Source: CAD feature listing. Evaluate the final solid. Frame: model axes, mm. Give positions to 0.01 mm unless a question says otherwise; leave off trailing zeros. Loops run counter-clockwise (first coordinate to the right, second up) from the corner with the lowest first, then second, coordinate; pieces in that order, holes last. Notation, with made-up numbers: M 69,49.5 L 114,49.5 A9 ccw 114,54.5 Z; hole C -8,-33 d10. An arc over 180 degrees is marked long. Answer in a Markdown table with one row per item.
```python
from build123d import *

# Parameters (mm, degrees)
ENL_V_MAT_EXTRU_1_DEPTH = 1


with BuildPart() as part:
    # Esquisse2 → Révolution2 (revolve)
    with BuildSketch(Plane.XY):
        with BuildLine():
            Line((-1.5, -3), (-1.5, -6))
            Line((-1.5, -6), (-4, -6))
            Line((-4, -6), (-4, 0))
            ThreePointArc((-4, 0), (-2.828427125, 2.828427125), (0, 4))
            Line((0, 4), (0, -3))
            Line((0, -3), (-1.5, -3))
        make_face()
    revolve(axis=Axis((0, 4, 0), (0, -1, 0)))

    # Esquisse3 → Enlèv. mat.-Extru.1 (cut)
    with BuildSketch(Plane.XZ.offset(6)):
        with BuildLine():
            add(Edge.make_bspline(
                [(-1.80863124, 2.541345123), (-1.808479721, 2.566576945), (-1.808185465, 2.615578129), (-1.805014729, 2.686862301), (-1.799544973, 2.753773198), (-1.792519265, 2.816312807), (-1.782799384, 2.874524095), (-1.771677826, 2.928435828), (-1.75798753, 2.978054639), (-1.741996794, 3.023469068), (-1.724042414, 3.06548569), (-1.704301487, 3.104630802), (-1.682899044, 3.141401404), (-1.659979633, 3.175784688), (-1.634459695, 3.207014642), (-1.607837422, 3.236160804), (-1.579113212, 3.262654216), (-1.548550296, 3.286362241), (-1.516934602, 3.307796564), (-1.483892299, 3.325862839), (-1.450188991, 3.341600286), (-1.415394884, 3.354330516), (-1.379762252, 3.364219477), (-1.343163483, 3.371125489), (-1.305772607, 3.375881264), (-1.280433508, 3.376250629), (-1.267698248, 3.376436269)],
                knots=[0, 0, 0, 0, 1.622528522, 3.151013738, 4.587225782, 5.939257941, 7.196658267, 8.381214254, 9.47772444, 10.503964975, 11.475138444, 12.414102326, 13.321377868, 14.209997518, 15.068075989, 15.912287155, 16.746865696, 17.577313739, 18.397854368, 19.200328723, 19.996378645, 20.787862277, 21.580050128, 22.371504404, 23.181529048, 24, 24, 24, 24], degree=3))
            add(Edge.make_bspline(
                [(-1.267698248, 3.376436269), (-1.253805469, 3.376070417), (-1.226383591, 3.37534829), (-1.185688202, 3.371418433), (-1.146357234, 3.363478815), (-1.107851049, 3.353522224), (-1.070793349, 3.339911348), (-1.034450069, 3.324259466), (-0.999939833, 3.304434891), (-0.966085568, 3.282749499), (-0.934048036, 3.25774196), (-0.903405408, 3.230569518), (-0.875113051, 3.200304639), (-0.848139657, 3.16798873), (-0.823868807, 3.132356169), (-0.800763662, 3.094654654), (-0.780305532, 3.05394524), (-0.760895229, 3.010948076), (-0.74421092, 2.964519866), (-0.729110025, 2.91492575), (-0.716872402, 2.861547844), (-0.706720882, 2.804552033), (-0.698897695, 2.743842361), (-0.693120072, 2.679563038), (-0.690103596, 2.611653966), (-0.689533129, 2.565198361), (-0.689240215, 2.541345123)],
                knots=[0, 0, 0, 0, 0.875057392, 1.727207867, 2.570264412, 3.399251263, 4.229017074, 5.053828049, 5.887584622, 6.731829445, 7.583639997, 8.443960147, 9.308026848, 10.190032267, 11.091770676, 12.020167189, 12.972467704, 13.958579741, 14.989078804, 16.076606933, 17.221320015, 18.435081626, 19.720875061, 21.074561036, 22.497895074, 24, 24, 24, 24], degree=3))
            add(Edge.make_bspline(
                [(-0.689240215, 2.541345123), (-0.689536199, 2.517598254), (-0.690112578, 2.471355268), (-0.693085762, 2.403758625), (-0.699013134, 2.339828893), (-0.706311275, 2.279386639), (-0.716548088, 2.222615428), (-0.729012582, 2.169485269), (-0.742990504, 2.11971682), (-0.760077838, 2.073746258), (-0.778998468, 2.030799872), (-0.799526075, 1.99045447), (-0.822133943, 1.952630546), (-0.847166636, 1.917738486), (-0.873431331, 1.884680376), (-0.902069059, 1.854605169), (-0.93255791, 1.826939612), (-0.96482414, 1.802036036), (-0.998498431, 1.779578013), (-1.033792029, 1.760620727), (-1.069815262, 1.743794249), (-1.107372434, 1.731042265), (-1.145702223, 1.720159494), (-1.185450047, 1.713129804), (-1.226246928, 1.70847555), (-1.253798722, 1.707844413), (-1.267698248, 1.707526012)],
                knots=[0, 0, 0, 0, 1.496607488, 2.914388442, 4.262485651, 5.541812885, 6.749953981, 7.895567619, 8.980172623, 10.005210728, 10.983286874, 11.936336572, 12.856292636, 13.757107149, 14.640766483, 15.514956722, 16.370989637, 17.232841377, 18.081413197, 18.918442167, 19.755471137, 20.583656588, 21.41504191, 22.264086897, 23.124254193, 24, 24, 24, 24], degree=3))
            add(Edge.make_bspline(
                [(-1.267698248, 1.707526012), (-1.28053559, 1.707744144), (-1.305960862, 1.708176169), (-1.343505356, 1.712413318), (-1.38007908, 1.719445505), (-1.415574616, 1.729301415), (-1.450241362, 1.741814634), (-1.483928981, 1.756972649), (-1.516416052, 1.775327151), (-1.54801261, 1.795949979), (-1.578259763, 1.819406928), (-1.6064329, 1.845919153), (-1.633209394, 1.874853048), (-1.658058785, 1.906520629), (-1.68153021, 1.940717467), (-1.70268935, 1.977765743), (-1.722416535, 2.017269766), (-1.740706112, 2.059533815), (-1.757219877, 2.105292204), (-1.770391091, 2.155440158), (-1.782811418, 2.209430466), (-1.79192615, 2.267809314), (-1.799834358, 2.33013628), (-1.804422361, 2.396815965), (-1.808343164, 2.467627223), (-1.808533454, 2.51632197), (-1.80863124, 2.541345123)],
                knots=[0, 0, 0, 0, 0.82614074, 1.636230647, 2.42850654, 3.22151677, 4.005075515, 4.799112676, 5.596456327, 6.404618302, 7.226350817, 8.05679228, 8.892237205, 9.761873943, 10.645770802, 11.559890835, 12.505927976, 13.487073095, 14.523090282, 15.633895838, 16.822583925, 18.088023083, 19.435493537, 20.865857947, 22.389433785, 24, 24, 24, 24], degree=3))
        make_face()
        with BuildLine():
            add(Edge.make_bspline(
                [(-1.605105599, 2.541981141), (-1.605023852, 2.520672046), (-1.604865594, 2.479419233), (-1.602515721, 2.419724601), (-1.599170136, 2.364139577), (-1.59416568, 2.312679231), (-1.587492401, 2.265267043), (-1.579593913, 2.22196849), (-1.570588452, 2.182700619), (-1.559609283, 2.147398904), (-1.547452492, 2.115233539), (-1.533935704, 2.085621273), (-1.519900759, 2.057891237), (-1.504090822, 2.032593058), (-1.487347707, 2.00938102), (-1.469369083, 1.988343478), (-1.450796759, 1.969019299), (-1.424302992, 1.947561621), (-1.390356536, 1.925127641), (-1.348216049, 1.905674198), (-1.305758021, 1.892833006), (-1.277113233, 1.891405835), (-1.262928115, 1.890699089)],
                knots=[0, 0, 0, 0, 1.564601651, 3.028951736, 4.386019676, 5.653114642, 6.824348509, 7.900668805, 8.88431448, 9.780488761, 10.613163047, 11.407444027, 12.169849642, 12.89344098, 13.595615509, 14.26934431, 14.924332585, 15.560171042, 16.769153194, 17.901006317, 18.960562374, 20, 20, 20, 20], degree=3))
            add(Edge.make_bspline(
                [(-1.262928115, 1.890699089), (-1.246853522, 1.891540168), (-1.214804369, 1.893217091), (-1.167603677, 1.905427209), (-1.122345984, 1.925920174), (-1.086485855, 1.949072591), (-1.05939208, 1.971591143), (-1.039825463, 1.990761174), (-1.02179068, 2.012163191), (-1.004765256, 2.035471294), (-0.989370848, 2.06106677), (-0.974527097, 2.088368697), (-0.961602786, 2.118032092), (-0.95413322, 2.138702882), (-0.950325451, 2.149240255)],
                knots=[0, 0, 0, 0, 1.331887272, 2.655486065, 4.012646414, 5.436183829, 6.178803566, 6.930724497, 7.703763371, 8.496530827, 9.320959298, 10.178042319, 11.071218497, 12, 12, 12, 12], degree=3))
            add(Edge.make_bspline(
                [(-0.950325451, 2.149240255), (-0.945737968, 2.163084868), (-0.936386065, 2.191308069), (-0.924669416, 2.235249723), (-0.914969473, 2.281357725), (-0.906617281, 2.329386525), (-0.90027545, 2.37957809), (-0.895891912, 2.431884075), (-0.893377451, 2.486304801), (-0.892971987, 2.523216067), (-0.892765856, 2.541981141)],
                knots=[0, 0, 0, 0, 0.877617242, 1.789083553, 2.735016418, 3.71249782, 4.722174671, 5.778575778, 6.870664861, 8, 8, 8, 8], degree=3))
            add(Edge.make_bspline(
                [(-0.892765856, 2.541981141), (-0.892815192, 2.560748136), (-0.892911405, 2.597346919), (-0.895770969, 2.650881984), (-0.899229308, 2.701840221), (-0.905195582, 2.750054281), (-0.911872778, 2.795764776), (-0.921031545, 2.838648534), (-0.930854849, 2.879133664), (-0.943127016, 2.916720139), (-0.956544156, 2.951787091), (-0.970695385, 2.984451245), (-0.985996373, 3.014738738), (-1.002854445, 3.04226954), (-1.020647463, 3.06749779), (-1.039441811, 3.090271765), (-1.05951754, 3.110463274), (-1.087584092, 3.133229632), (-1.123765401, 3.156924472), (-1.169007106, 3.178189343), (-1.215723695, 3.190725625), (-1.247275437, 3.192421751), (-1.262928115, 3.193263192)],
                knots=[0, 0, 0, 0, 1.353201578, 2.638969622, 3.865559904, 5.035676431, 6.141732754, 7.195734042, 8.19695873, 9.144657206, 10.044788335, 10.904062871, 11.710933862, 12.489720227, 13.229995877, 13.935715626, 14.616825307, 15.279494989, 16.538995736, 17.725922936, 18.871840505, 20, 20, 20, 20], degree=3))
            add(Edge.make_bspline(
                [(-1.262928115, 3.193263192), (-1.277109142, 3.192542637), (-1.305847895, 3.191082387), (-1.348370358, 3.178419537), (-1.390359144, 3.158811848), (-1.424078124, 3.13636234), (-1.450352786, 3.114927418), (-1.469178663, 3.096042766), (-1.486571406, 3.074886349), (-1.503356006, 3.051861153), (-1.518682213, 3.02639658), (-1.533568016, 2.998957155), (-1.546683445, 2.96908953), (-1.559017747, 2.936899522), (-1.569881275, 2.90153329), (-1.579275962, 2.86232535), (-1.587671251, 2.819074671), (-1.593721707, 2.771566799), (-1.598807927, 2.720028274), (-1.602614415, 2.664356134), (-1.604836941, 2.604541443), (-1.605014092, 2.563289689), (-1.605105599, 2.541981141)],
                knots=[0, 0, 0, 0, 1.039778295, 2.107176824, 3.232337611, 4.43520669, 5.071253539, 5.720927637, 6.389866065, 7.081397607, 7.811854436, 8.571243718, 9.372887587, 10.205834777, 11.102302774, 12.088086757, 13.166194718, 14.33675119, 15.604261439, 16.970055543, 18.43488556, 20, 20, 20, 20], degree=3))
        make_face(mode=Mode.SUBTRACT)
    extrude(amount=-ENL_V_MAT_EXTRU_1_DEPTH, mode=Mode.SUBTRACT)


solid = part.part
```
Q1. Ray query, probe 1 along Z at (x, y) = (0, -4.6); probe 2 along X at (y, z) = (-5.5, -0.5). Return the intervals inside material, ascending. Write a range as from..to.
Values follow:
| item | result |
|---|---|
| probe 1 | -4..-1.5, 1.5..4 |
| probe 2 | -3.97..-1.41, 1.41..3.97 |
Q2. Section query A-A (z = 0). Output: boundary loops of the cut face in (x, y), plus the area to 3 significant figures.
Values follow:
| item | result |
|---|---|
| outline | M -4,-6 L -1.5,-6 L -1.5,-3 L 1.5,-3 L 1.5,-6 L 4,-6 L 4,0 A4 ccw -4,0 Z |
| area | 64.1 mm^2 |
Q3. Contact query for flat-ended pins moving along their axis: pin 1 Ø2.5 at (x, z) = (0, 0) entering from -Y; pin 2 Ø1 at (y, z) = (-1, 2) entering from -X. Output: stop coordinate, or through.
Values follow:
| item | result |
|---|---|
| pin 1 | y = -3 |
| pin 2 | x = -3.71 |
Q4. Section query D-D (z = -2.5). Output: boundary loops of the cut face in (x, y) (1 decimal).
Values follow:
| item | result |
|---|---|
| outline | M -3.1,-6 L 3.1,-6 L 3.1,0 A3.1 ccw -3.1,0 Z |
Q5. Mould query, pull axis X, two halves, no side actions, for faces 1 (the cylindrical face through (0.867, -2.958, 3.905)), 2 (the flat face through (2, -6, 0)), 3 (the flat face through (0, -3, 0)). Classes: +X half, -X half, draft (parallel to the pull), parting line (faces both ways), or undercut.
Values follow:
| item | result |
|---|---|
| face 1 | parting line |
| face 2 | draft |
| face 3 | undercut |
Q6. Section query C-C (y = -1.5). Output: boundary loops of the cut face in (x, z).
Values follow:
| item | result |
|---|---|
| outline | C 0,0 d8 |
Q7. Section query B-B (x = 0). Output: boundary loops of the cut face in (y, z), plus the area to 3 significant figures.
Values follow:
| item | result |
|---|---|
| outline | M -6,-4 L 0,-4 A4 ccw 0,4 L -6,4 L -6,1.5 L -3,1.5 L -3,-1.5 L -6,-1.5 Z |
| area | 64.1 mm^2 |
